Geometry: see drawing. Coordinates: mm, zero at the bounding-box minimum. A direction names the side the tool comes from. Give positions to 0.01 mm unless a question says otherwise; leave off trailing zeros. Write each loop counter-clockwise with the first axis right and the second up, starting at its lowest first coordinate (ties: lowest second). Pieces come first, ordered by that corner, then holes. Notation, with made-up numbers: (50.25, 22.25) -> (84.25, 22.25) arc R29 ccw to (84.25, 45.25) -> close; hole circle Ø6 at (39, 68.25). An arc over 180 degrees is marked (long way). Use CSV: the item, a comma, the result in double quotes. Start each with the question number.
1) Set-up query: the marked faces 4 and 5. Return all of +Z, -Z, +X, -X, +Y, -Y with unobstructed straight access to the full face (end or side cutting, diameter ignored); none if empty.
2) Contact query for flat-ended pins moving along their axis: P1, Ø3, axis at x = 118, z = 55.5, coming from the +Y side; P2, Ø2.5, axis at x = 20, y = 19, coming from the -Z side. Output: stop coordinate, or through.
3) Draft query along X for the marked faces 1, 2 and 3. Return one class per face: pulls with the +X half, pulls with the -X half, needs draft (parallel to the pull), parting line crosses it, or undercut.
4) Material intervals for line 1 (Z direction, x = 26.5, y = 20); line 2 (X direction, y = 7, z = 59); line 3 (X direction, y = 19, z = 1), sorted ascending. Write a range as [from, to].
5) Section B-B (x = 20). Output: boundary loops of the cut face in (y, z), plus the area to 3 significant figures.
6) Section A-A (y = 19). Output: boundary loops of the cut face in (x, z).
7) Section D-D (y = 7). Output: boundary loops of the cut face in (x, z).
8) Section C-C (z = 10.5). Output: boundary loops of the cut face in (x, y).
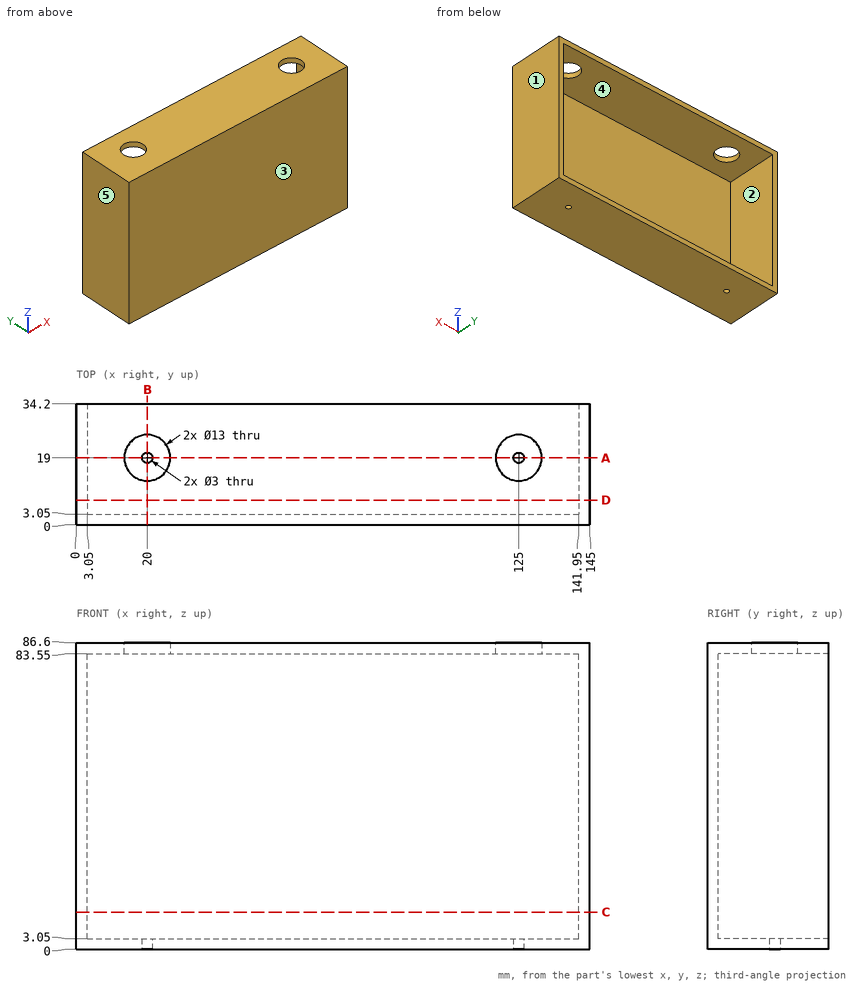
Answers follow:
1,face 4,"+Y"
1,face 5,"+Z, -Z, -X, +Y, -Y"
2,P1,"stops at y = 3.05"
2,P2,"passes through"
3,face 1,"pulls with the +X half"
3,face 2,"undercut"
3,face 3,"needs draft"
4,line 1,"z = [0, 3.05], [83.55, 86.6]"
4,line 2,"x = [0, 3.05], [141.95, 145]"
4,line 3,"x = [0, 18.5], [21.5, 123.5], [126.5, 145]"
5,outline,"(0, 0) -> (17.5, 0) -> (17.5, 3.05) -> (3.05, 3.05) -> (3.05, 83.55) -> (12.5, 83.55) -> (12.5, 86.6) -> (0, 86.6) -> close; (20.5, 0) -> (34.2, 0) -> (34.2, 3.05) -> (20.5, 3.05) -> close; (25.5, 83.55) -> (34.2, 83.55) -> (34.2, 86.6) -> (25.5, 86.6) -> close"
5,area,"405 mm^2"
6,outline,"(0, 0) -> (18.5, 0) -> (18.5, 3.05) -> (3.05, 3.05) -> (3.05, 83.55) -> (13.5, 83.55) -> (13.5, 86.6) -> (0, 86.6) -> close; (21.5, 0) -> (123.5, 0) -> (123.5, 3.05) -> (21.5, 3.05) -> close; (26.5, 83.55) -> (118.5, 83.55) -> (118.5, 86.6) -> (26.5, 86.6) -> close; (126.5, 0) -> (145, 0) -> (145, 86.6) -> (131.5, 86.6) -> (131.5, 83.55) -> (141.95, 83.55) -> (141.95, 3.05) -> (126.5, 3.05) -> close"
7,outline,"(0, 0) -> (145, 0) -> (145, 86.6) -> (0, 86.6) -> close; hole (3.05, 3.05) -> (141.95, 3.05) -> (141.95, 83.55) -> (3.05, 83.55) -> close"
8,outline,"(0, 0) -> (145, 0) -> (145, 34.2) -> (141.95, 34.2) -> (141.95, 3.05) -> (3.05, 3.05) -> (3.05, 34.2) -> (0, 34.2) -> close"
